Geometry check sheet. Reference: drawing and pictorial views, mm from the part's lowest x, y, z. A direction names the side the tool comes from. Give positions to 0.01 mm unless a question says otherwise; leave off trailing zeros. Order: outer loops, then holes, each group sorted by start corner. A loop starts at its lowest first (then second) coordinate and runs counter-clockwise, first axis right, second up. Notation, with made-up numbers: M 23.25,60 L 68.25,60 A11 cw 68.25,73 Z; hole C 38.5,75.25 d2. An arc over 180 degrees is marked long. Answer as a JSON object with one key per item and string values. Group by question number.
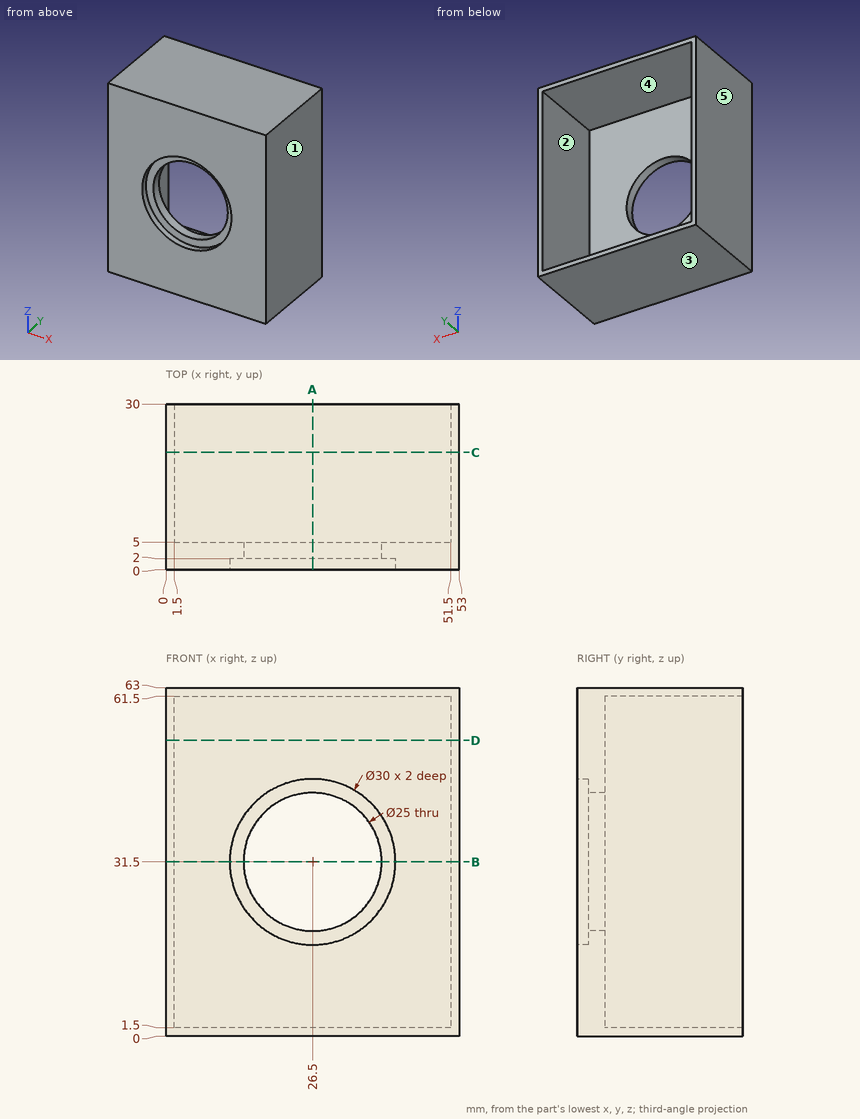
1. Cross-section at B-B (z = 31.5). Record the cut outline in (x, y), and give its area (3 significant figures).
2. Release check for a two-part mould opening along X. For the marked faces 1, 2 and 3 record: released by +X, released by -X, zero draft, split by the parting line, or undercut.
3. Cross-section at D-D (z = 53.5). Record the cut outline in (x, y), and give its area (3 significant figures).
4. Cross-section at C-C (y = 21.25). Record the cut outline in (x, z).
5. Access from +Z, -Z, +X, -X, +Y, -Y to the whole of each face (thin tool, end or side, straight path). Record for the marked faces 4 and 5.
6. Depth check by flat-ended pin: pin 1 (25 mm diameter, centred on x = 33, z = 40, fed in from +Y). Enter the tip coordinate at first touch or a pass-through.
7. Thickness scan on line 1 along Z through (x, y) = (26.5, 2.8); line 2 along X through (y, z) = (21, 59); line 3 along Z through (x, y) = (26.5, 1.4). Record the ranges inside material, lowest first. Write a range as [from, to].
8. Cross-section at A-A (x = 26.5). Record the cut outline in (y, z).
Report:
{
 "1": {"outline": "M 0,0 L 11.5,0 L 11.5,2 L 14,2 L 14,5 L 1.5,5 L 1.5,30 L 0,30 Z; M 39,2 L 41.5,2 L 41.5,0 L 53,0 L 53,30 L 51.5,30 L 51.5,5 L 39,5 Z", "area": "205 mm2"},
 "2": {"face 1": "released by +X", "face 2": "undercut", "face 3": "zero draft"},
 "3": {"outline": "M 0,0 L 53,0 L 53,30 L 51.5,30 L 51.5,5 L 1.5,5 L 1.5,30 L 0,30 Z", "area": "340 mm2"},
 "4": {"outline": "M 0,0 L 53,0 L 53,63 L 0,63 Z; hole M 1.5,1.5 L 51.5,1.5 L 51.5,61.5 L 1.5,61.5 Z"},
 "5": {"face 4": "+Y", "face 5": "+Z, -Z, -X, +Y, -Y"},
 "6": {"pin 1": "stops at y = 5"},
 "7": {"line 1": "z = [0, 19], [44, 63]", "line 2": "x = [0, 1.5], [51.5, 53]", "line 3": "z = [0, 16.5], [46.5, 63]"},
 "8": {"outline": "M 0,0 L 30,0 L 30,1.5 L 5,1.5 L 5,19 L 2,19 L 2,16.5 L 0,16.5 Z; M 0,46.5 L 2,46.5 L 2,44 L 5,44 L 5,61.5 L 30,61.5 L 30,63 L 0,63 Z"}
}
